Can you work these out from the model? Positions are in its coordinate system, mm. A direction names the side the tool comes from. Coordinates: 2 decimals unless noted, no trailing zeros. Write each loop counter-clockwise with the first axis right and the second up, starting at its lowest first coordinate (ties: lowest second). Pieces come first, ordered by that corner, then holes. Notation, with made-up numbers: M 45,29 L 83,29 A35 cw 83,67 Z; hole C -18,85.25 d7. An arc over 180 degrees is marked long. Answer as a JSON object with one key per item and string values. Group by question number.
from build123d import *

# Parameters (mm, degrees)
EXTRUDE_1_DEPTH     = 25
SKETCH_2_R          = 1.5
CUT_EXTRUDE_1_DEPTH = 10
SKETCH_3_R          = 1.5
CUT_EXTRUDE_2_DEPTH = 10


with BuildPart() as part:
    # 草图1 → 凸台-拉伸1 (new body)
    with BuildSketch(Plane(origin=(0, 0, 0), x_dir=(1, 0, 0), z_dir=(0, 1, 0))):
        Polygon((0, 0), (25, 0), (25, 5), (5, 5), (5, 25), (0, 25), align=None)
    extrude(amount=EXTRUDE_1_DEPTH)

    # 草图2 → 切除-拉伸1 (cut)
    with BuildSketch(Plane(origin=(0, 0, -5), x_dir=(-1, 0, 0), z_dir=(0, 0, -1))):
        with Locations((-20, 20)):
            Circle(SKETCH_2_R)
        with Locations((-20, 5)):
            Circle(SKETCH_2_R)
    extrude(amount=-CUT_EXTRUDE_1_DEPTH, mode=Mode.SUBTRACT)

    # 草图3 → 切除-拉伸2 (cut)
    with BuildSketch(Plane(origin=(5, 0, 0), x_dir=(0, 0, -1), z_dir=(1, 0, 0))):
        with Locations((20, 20)):
            Circle(SKETCH_3_R)
        with Locations((20, 5.070253282)):
            Circle(SKETCH_3_R)
    extrude(amount=-CUT_EXTRUDE_2_DEPTH, mode=Mode.SUBTRACT)


solid = part.part
Q1. We'd pull the mould along X, two halves only. Please class faces 3 (the flat face through (7, 25, -4)), 4 (the flat face through (5, 12, -15)), 5 (the cylindrical face through (21.11, 21.01, -2.54)), 6 (the cylindrical face through (21.5, 5.07, -2.54)): pulls with the +X half, pulls with the -X half, needs draft (parallel to the pull), parting line crosses it, or undercut.
Q2. Please list where these lines run through material, in increasing order: L1, parallel to Y at x = 20, z = -0.95; L2, parallel to Y at x = 2.15, z = -20; L3, parallel to X at y = 6.75, z = -6.5.
Q3. If we section it at A-A on x = 20: List the corners of the cut face in (y, z) for me, and give its area (3 significant figures).
Q4. If we section it at D-D on z = -3.75: List the corners of the cut face in (x, y) for me.
Q5. Will these pins go through, and if not, where does the flat tip stop? pin 1 (2.5 mm diameter, centred on x = 20, y = 5, fed in from -Z); pin 2 (4 mm diameter, centred on y = 20, z = -20, fed in from +X); pin 3 (8 mm diameter, centred on x = 17.5, y = 3.5, fed in from -Z).
Q6. If we section it at B-B on y = 20: List the corners of the cut face in (x, z) for me, and give its area (3 significant figures).
Q7. If we section it at C-C on z = -20: List the corners of the cut face in (x, y) for me.
Q8. On a 3-axis mill with a long thin cutter (end or side, diameter ignored), from which of +Z, -Z, +X, -X, +Y, -Y can I reach the whole of each face in a straight line? I mean faces 1 (the flat face through (15, 12, -5)), 2 (the flat face through (0, 12, -13)). Say none if no direction works.
Reply:
{
 "1": {"face 3": "needs draft", "face 4": "pulls with the +X half", "face 5": "undercut", "face 6": "undercut"},
 "2": {"L1": "0 to 3.5, 6.5 to 18.5, 21.5 to 25", "L2": "0 to 3.57, 6.57 to 18.5, 21.5 to 25", "L3": "0 to 5"},
 "3": {"outline": "M 0,-5 L 3.5,-5 L 3.5,0 L 0,0 Z; M 6.5,-5 L 18.5,-5 L 18.5,0 L 6.5,0 Z; M 21.5,-5 L 25,-5 L 25,0 L 21.5,0 Z", "area": "95.0 mm^2"},
 "4": {"outline": "M 0,0 L 25,0 L 25,25 L 0,25 Z; hole C 20,5 d3; hole C 20,20 d3"},
 "5": {"pin 1": "through", "pin 2": "x = 5", "pin 3": "z = -5"},
 "6": {"outline": "M 0,-25 L 5,-25 L 5,-21.5 L 0,-21.5 Z; M 0,-18.5 L 5,-18.5 L 5,-5 L 18.5,-5 L 18.5,0 L 0,0 Z; M 21.5,-5 L 25,-5 L 25,0 L 21.5,0 Z", "area": "195 mm^2"},
 "7": {"outline": "M 0,0 L 5,0 L 5,3.57 L 0,3.57 Z; M 0,6.57 L 5,6.57 L 5,18.5 L 0,18.5 Z; M 0,21.5 L 5,21.5 L 5,25 L 0,25 Z"},
 "8": {"face 1": "-Z, +X, +Y, -Y", "face 2": "+Z, -Z, -X, +Y, -Y"}
}
